Job drawing, mm, ordinate dimensions from the low corner. One solid piece. Give positions to 0.01 mm unless a question says otherwise; leave off trailing zeros. Order: outer loops, then holes, each group sorted by start corner. A loop starts at its lowest first (then second) coordinate and runs counter-clockwise, first axis right, second up. Notation, with made-up numbers: (0.5, 65) -> (4.5, 65) arc R3 cw to (4.5, 69) -> close; hole circle Ø10 at (1.5, 44). An arc over 180 degrees is marked (long way). Use CSV: the item, a comma, the result in double quotes. Start each with the question number.
1. Wall check: line 1 (X direction, y = 6.75, z = 39); line 2 (Y direction, x = 6.25, z = 29); line 3 (X direction, y = 8.25, z = 44.5). Give the ranges that are in metal, low to high. Write a range as from..to.
2. Cut at A-A on x = 6.35. List the corners of the cut face in (y, z), then the cut area to 3 significant figures.
3. Drop flat-ended pins along their axis: pin 1 (1.1 mm diameter, centred on y = 11.5, z = 37, fed in from +X); pin 2 (3 mm diameter, centred on x = 10, z = 33, fed in from -Y) (1 decimal); pin 3 (2.5 mm diameter, centred on x = 6.5, z = 37.5, fed in from +Y). Give the stop position or say it passes through.
4. Cut at B-B on z = 40. List the corners of the cut face in (x, y).
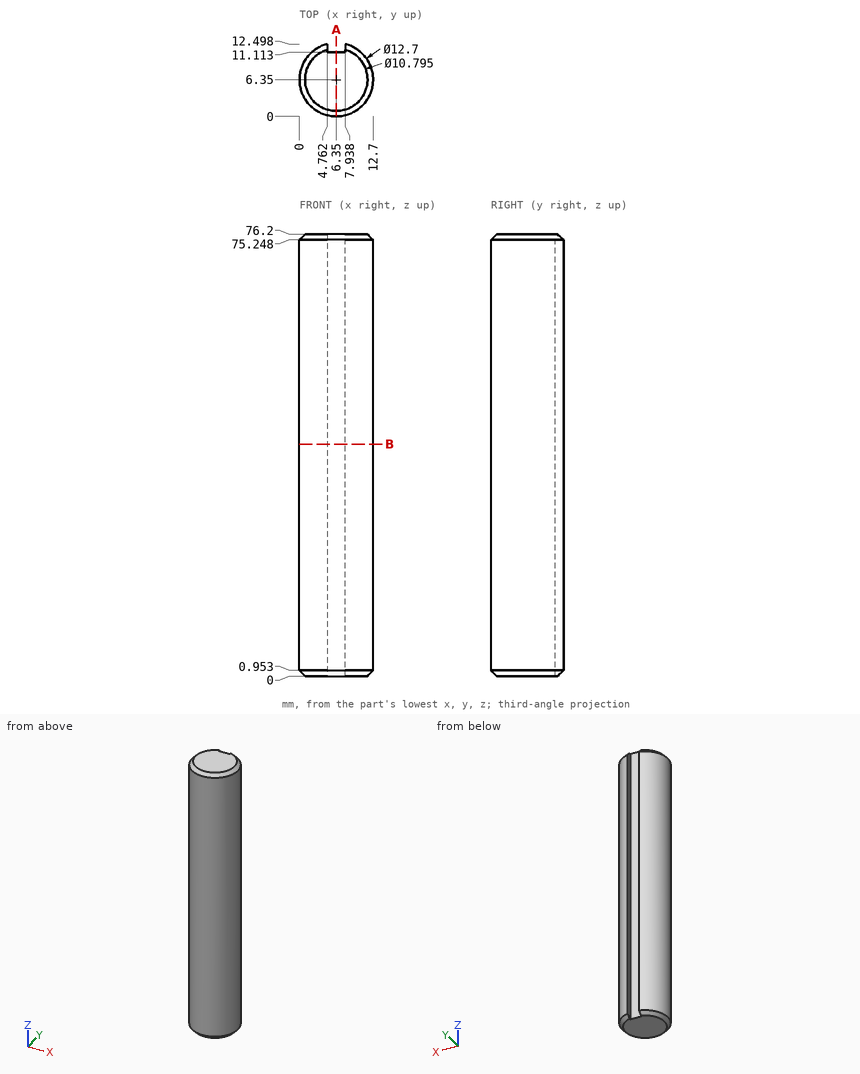
Verdict:
1,line 1,"0.01..12.69"
1,line 2,"0..11.11"
1,line 3,"0.29..12.41"
2,outline,"(0, 0.95) -> (0.95, 0) -> (11.11, 0) -> (11.11, 76.2) -> (0.95, 76.2) -> (0, 75.25) -> close"
2,area,"846 mm^2"
3,pin 1,"x = 10.73"
3,pin 2,"y = 0.4"
3,pin 3,"y = 11.11"
4,outline,"(4.76, 11.11) -> (4.76, 12.5) arc R6.35 ccw (long way) to (7.94, 12.5) -> (7.94, 11.11) -> close"
